CAD build for the part. Positions are in the model's coordinates, mm. A direction names the side the tool comes from. Round coordinates to 2 decimals unless told otherwise and drop trailing zeros. Write each loop counter-clockwise with the first axis right and the second up, starting at its lowest first coordinate (ties: lowest second). Pieces come first, ordered by that corner, then holes. Notation, with made-up numbers: (2.25, -21) - (47.25, -21) arc R22 cw to (47.25, 5) - close; hole circle Ø1 at (-8, 24). An arc over 180 degrees is marked (long way). Answer in a Markdown table with one row per item.
```python
from build123d import *

# Parameters (mm, degrees)
F0_W     = 127
F0_H     = 127
F1_DEPTH = 101.6
F3_DEPTH = 76.2
F5_DEPTH = 76.2
F7_R     = 8.382674823
F8_DEPTH = 50.8
F6_R     = 7.7668100233
F9_DEPTH = 50.8
F10_R    = 5.08


with BuildPart() as f1:
    # F0 (on Front) → F1 (new body)
    with BuildSketch(Plane.XZ):
        Rectangle(F0_W, F0_H)
    extrude(amount=F1_DEPTH)

    # F2 (on face) → F3 (cut)
    with BuildSketch(Plane.XY.offset(63.5)):
        Polygon((-12.7, 0), (-63.5, 0), (-63.5, -50.8), align=None)
    extrude(amount=-F3_DEPTH, mode=Mode.SUBTRACT)

    # F4 (on face) → F5 (cut)
    with BuildSketch(Plane.XY.offset(63.5)):
        Polygon((12.7, -101.6), (63.5, -101.6), (63.5, -50.8), align=None)
    extrude(amount=-F5_DEPTH, mode=Mode.SUBTRACT)

    # F7 (on face) → F8 (cut)
    with BuildSketch(Plane.XY.offset(-12.7)):
        with Locations((-48.26, -15.24)):
            Circle(F7_R)
    extrude(amount=-F8_DEPTH, mode=Mode.SUBTRACT)

    # F6 (on face) → F9 (cut)
    with BuildSketch(Plane.XY.offset(-12.7)):
        with Locations((47.7252677083, -86.36)):
            Circle(F6_R)
    extrude(amount=-F9_DEPTH, mode=Mode.SUBTRACT)

    # F10
    f10_edges = [f1.edges().sort_by_distance(p)[0] for p in [
        (-38.1, -25.4, 63.5),
        (-63.5, -76.2, 63.5),
        (-25.4, -101.6, 63.5),
        (38.1, -76.2, 63.5),
        (25.4, 0, 63.5),
        (63.5, -25.4, 63.5),
        (63.5, -50.8, 25.4),
        (63.5, 0, 0),
        (63.5, -50.8, -63.5),
        (63.5, -76.2, -12.7),
        (38.1, -101.6, -12.7),
        (12.7, -101.6, 25.4),
        (-63.5, -101.6, 0),
        (0, -101.6, -63.5),
        (-63.5, -50.8, -63.5),
        (-63.5, -50.8, 25.4),
        (-63.5, -25.4, -12.7),
        (0, 0, -63.5),
        (-38.1, 0, -12.7),
        (-12.7, 0, 25.4),
    ]]
    fillet(f10_edges, radius=F10_R)


solid = f1.part
```
Q1. 3-axis set-ups, long thin cutter, end or side, ignore diameter. For faces 1 (the cylindrical face through (62.051, -74.778, -14.228)), 2 (the cylindrical face through (61.972, -1.449, 0.818)), 3 (the flat face through (-38.4, -25.7, 22.6)): which of +Z, -Z, +X, -X, +Y, -Y reach the whole face in a straight line?
Computed:
| item | result |
|---|---|
| face 1 | +Z, +X, -Y |
| face 2 | +Z, -Z, +X, +Y |
| face 3 | +Z, -X, +Y |
Q2. Saw through at A-A on z = -21.5. List the corners of the cut face in (x, y), then the cut area to 3 significant figures.
Computed:
| item | result |
|---|---|
| outline | (-63.5, -96.52) arc R5.08 ccw to (-58.42, -101.6) - (63.5, -101.6) - (63.5, -5.08) arc R5.08 ccw to (58.42, 0) - (-63.5, 0) - close; hole circle Ø16.77 at (-48.26, -15.24); hole circle Ø15.53 at (47.73, -86.36) |
| area | 12,500 mm2 |
Q3. Pull direction Y, two halves, no side cores. Call faces 4 (the flat face through (38.4, -75.9, 22.6)), 5 (the flat face through (41, -79, -12.7)), 6 (the cylindrical face through (42, -81.11, -37.74)), 7 (the flat face through (10, 0, -12)): released by +Y, released by -Y, zero draft, split by the parting line, or undercut.
Computed:
| item | result |
|---|---|
| face 4 | released by -Y |
| face 5 | zero draft |
| face 6 | undercut |
| face 7 | released by +Y |
Q4. Flat gauge pin, fed straight in: pin 1 (6 mm diameter, centred on x = 37.5, z = 18, fed in from -Y). Where does the tip first touch, or does it go through?
Computed:
| item | result |
|---|---|
| pin 1 | stops at y = -79.8 |
Q5. Drill centre lines: line 1 (Y direction, x = -48.26, z = -43.5); line 2 (X direction, y = -86, z = -46); line 3 (Z direction, x = -35, y = -11.5). Where is each one in solid material? Low to high.
Computed:
| item | result |
|---|---|
| line 1 | y = -101.6 to -23.62, -6.86 to 0 |
| line 2 | x = -63.5 to 39.97, 55.48 to 63.5 |
| line 3 | z = -63.5 to -12.7 |
